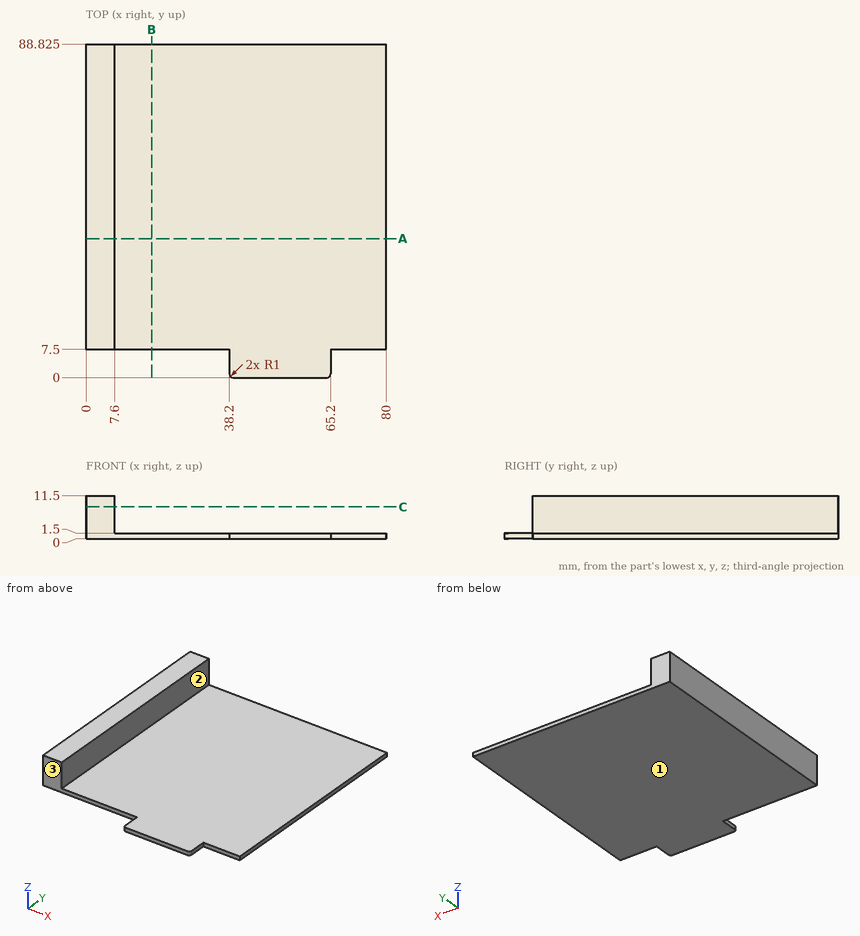
Print and shaded views of the part. All mm, measured from the part's lowest x, y and z. A direction names the side the tool comes from. Coordinates: 2 decimals unless noted, no trailing zeros. Order: outer loops, then holes, each group sorted by start corner. A loop starts at its lowest first (then second) coordinate and runs counter-clockwise, first axis right, second up. Notation, with made-up numbers: M 65,72.5 L 85,72.5 A29 cw 85,101.5 Z; hole C -33.75,-31.75 d2. An arc over 180 degrees is marked long. One line per question, with ' | ' between items. Start each with the question number.
Q1. Saw through at C-C (z = 8.5). List the corners of the cut face in (x, y) (3 decimals).
Q2. 3-axis set-ups, long thin cutter, end or side, ignore diameter. For the marked faces 1, 2 and 3: which of +Z, -Z, +X, -X, +Y, -Y reach the whole face in a straight line?
Q3. Saw through at B-B (x = 17.5). List the corners of the cut face in (y, z) (3 decimals), then the cut area to 3 significant figures.
Q4. Probe L1, parallel to Y at x = 24, z = 0.75 (3 decimals); L2, parallel to X at y = 17.5, z = 10.25; L3, parallel to Z at x = 43.5, y = 80.5. List the from-to ranges inside material, lowest first. Write a range as from..to.
Q5. Flat gauge pins, fed straight in: pin 1 Ø1.2 at (x, z) = (74.5, 1) entering from -Y; pin 2 Ø0.8 at (y, z) = (2.5, 0.5) entering from -X; pin 3 Ø5 at (y, z) = (66, 5.5) entering from +X. Where does each tip first touch, or does it go through?
Q6. Saw through at A-A (y = 37). List the corners of the cut face in (x, z), then the cut area to 3 significant figures.
Check values:
1) outline: M 0,7.5 L 7.6,7.5 L 7.6,88.825 L 0,88.825 Z
2) face 1: -Z, +X, -X, +Y, -Y | face 2: +Z, +X, +Y, -Y | face 3: +Z, -Z, -X, -Y
3) outline: M 7.5,0 L 88.825,0 L 88.825,1.5 L 7.5,1.5 Z | area: 122 mm2
4) L1: y = 7.5..88.825 | L2: x = 0..7.6 | L3: z = 0..1.5
5) pin 1: stops at y = 7.5 | pin 2: stops at x = 38.2 | pin 3: stops at x = 7.6
6) outline: M 0,0 L 80,0 L 80,1.5 L 7.6,1.5 L 7.6,11.5 L 0,11.5 Z | area: 196 mm2
